```python
from build123d import *

# Parameters (mm, degrees)
CYLINDER001_R     = 4.5
CYLINDER001_DEPTH = 15
CYLINDER_R        = 5
CYLINDER_DEPTH    = 15


with BuildPart() as cilindre001:
    # Cylinder001 → Cylinder001 (new body)
    with BuildSketch(Plane.XY):
        Circle(CYLINDER001_R)
    extrude(amount=CYLINDER001_DEPTH)


with BuildPart() as cut:
    # Cylinder → Cylinder (new body)
    with BuildSketch(Plane.XY):
        Circle(CYLINDER_R)
    extrude(amount=CYLINDER_DEPTH)

    # Cut: cut Cilindre001
    add(cilindre001.part, mode=Mode.SUBTRACT)


with BuildPart() as con001:
    # Cone001 → Cone001 (revolve)
    with BuildSketch(Plane(origin=(0, 0, 15), x_dir=(1, 0, 0), z_dir=(0, -1, 0))):
        Polygon((0, 0), (4.5, 0), (24, 30), (0, 30), align=None)
    revolve(axis=Axis((0, 0, 15), (0, 0, 1)))


with BuildPart() as fusion:
    # Cone → Cone (revolve)
    with BuildSketch(Plane(origin=(0, 0, 15), x_dir=(1, 0, 0), z_dir=(0, -1, 0))):
        Polygon((0, 0), (5, 0), (25, 30), (0, 30), align=None)
    revolve(axis=Axis((0, 0, 15), (0, 0, 1)))

    # Cut001: cut Con001
    add(con001.part, mode=Mode.SUBTRACT)

    # Fusion: union Cut
    add(cut.part)


solid = fusion.part
```
Geometry check sheet. Reference: the model listing, model coordinates, mm. A direction names the side the tool comes from. Round coordinates to 2 decimals unless told otherwise and drop trailing zeros. Write each loop counter-clockwise with the first axis right and the second up, starting at its lowest first coordinate (ties: lowest second). Pieces come first, ordered by that corner, then holes. Notation, with made-up numbers: (-32.75, -29) -> (-17.75, -29) arc R25 ccw to (-17.75, 10) -> close; hole circle Ø2 at (-24, 53.25). An arc over 180 degrees is marked (long way). Put each result on its own line as item: value.
1) Cross-section at A-A, the plane y = 0. Enter the section's corners in (x, z), plus the area to 3 significant figures.
Recorded:
outline: (-25, 45) -> (-5, 15) -> (-5, 0) -> (-4.5, 0) -> (-4.5, 15) -> (-24, 45) -> close; (4.5, 0) -> (5, 0) -> (5, 15) -> (25, 45) -> (24, 45) -> (4.5, 15) -> close
area: 60.0 mm2
2) Cross-section at C-C, the plane z = 9. Enter the section's corners in (x, y).
Recorded:
outline: circle Ø10 at (0, 0); hole circle Ø9 at (0, 0)
3) Release check for a two-part mould opening along Y. For faces 1 (the face through (-2.32, -10.44, 23.54)), 2 (the face through (-9.4, 22.3, 45)), 3 (the face through (4.639, -8.919, 23.543)) record: pulls with the +Y half, pulls with the -Y half, needs draft (parallel to the pull), parting line crosses it, or undercut.
Recorded:
face 1: parting line crosses it
face 2: needs draft
face 3: undercut
4) Thickness scan on probe 1 along Y at (x, z) = (0, 11); probe 2 along Y at (x, z) = (-2, 29.5); probe 3 along X at (y, z) = (15, 43). Record the ranges inside material, lowest first. Write a range as from..to.
Recorded:
probe 1: y = -5..-4.5, 4.5..5
probe 2: y = -14.53..-13.78, 13.78..14.53
probe 3: x = -18.31..-17.04, 17.04..18.31
5) Depth check by flat-ended pin: P1, Ø8, axis at x = 13, y = -18, coming from the +Z side; P2, Ø3, axis at x = -16.5, y = -3, coming from the +Z side; P3, Ø2, axis at x = -1.5, z = 19.5, coming from the +Y side; P4, Ø1.5, axis at y = -4.5, z = 31, coming from the -X side. Enter the tip coordinate at first touch or a pass-through.
Recorded:
P1: stops at z = 45
P2: stops at z = 36.19
P3: stops at y = 8.56
P4: stops at x = -15.57
6) Access from +Z, -Z, +X, -X, +Y, -Y to the whole of each face (thin tool, end or side, straight path). Record for faces 4 (the face through (-1.08, -4.88, 7.4)), 5 (the face through (-0.59, 4.46, 7.4)).
Recorded:
face 4: -Z
face 5: +Z, -Z
7) Cross-section at D-D, the plane z = 35. Enter the section's corners in (x, y), plus the area to 3 significant figures.
Recorded:
outline: circle Ø36.67 at (0, 0); hole circle Ø35 at (0, 0)
area: 93.8 mm2
